Build history of the part. All positions in model axes, mm. Face numbers are marked on the shaded views. A direction names the side the tool comes from. Round coordinates to 2 decimals unless told otherwise and drop trailing zeros. Write each loop counter-clockwise with the first axis right and the second up, starting at its lowest first coordinate (ties: lowest second). Pieces come first, ordered by that corner, then holes. Notation, with made-up numbers: (86.25, 41) - (103.25, 41) arc R18 cw to (103.25, 56) - close; hole circle Ø5 at (78.5, 57). An arc over 180 degrees is marked (long way). Answer as a JSON object with one key per item and string values. Group by question number.
Item 1: Flat gauge pins, fed straight in: pin 1 (1.5 mm diameter, centred on x = 5.5, z = -0.5, fed in from +Y); pin 2 (1 mm diameter, centred on x = 5, y = 1, fed in from +Z). Where does each tip first touch, or does it go through?
Item 2: Slice it at A-A, the plane x = 7.75. List the corners of the cut face in (y, z), then the cut area to 3 significant figures.
Item 3: Probe line 1 (X direction, y = 1, z = -2.25); line 2 (X direction, y = -3, z = -0.25); line 3 (Y direction, x = 5.75, z = 0). List the from-to ranges inside material, lowest first. Write a range as from..to.
Item 4: Which spindle directions (+Z, -Z, +X, -X, +Y, -Y) get a long thin tool onto all of the face, cutting with end or side? Do the marked faces 1 and 2. Say none if no direction does.
from build123d import *

# Parameters (mm, degrees)
CUT_EXTRUDE_1_DEPTH = 1.53
CUT_EXTRUDE_1_TAPER = 10
FILLET_1_R          = 0.1


with BuildPart() as part:
    # Sketch 1 → Revolve 892 (revolve)
    with BuildSketch(Plane.XY, mode=Mode.PRIVATE) as revolve_892_sk:
        with BuildLine():
            Line((-2.162677546, 2.622032296), (-0.7, 2.75))
            Line((-0.7, 2.75), (-0.7, 3.25))
            Line((-0.7, 3.25), (0, 3.25))
            Line((0, 3.25), (0, 1.2))
            Line((0, 1.2), (0.5, 1.2))
            Line((0.5, 1.2), (0.5, 1.5))
            Line((0.5, 1.5), (10, 1.5))
            Line((10, 1.5), (10, 0))
            Line((10, 0), (-3.3, 0))
            ThreePointArc((-3.3, 0), (-3.234218103, 0.957402372), (-3.038108771, 1.896810531))
            ThreePointArc((-3.038108771, 1.896810531), (-2.713468973, 2.395917729), (-2.162677546, 2.622032296))
        make_face()
    revolve(revolve_892_sk.sketch.rotate(Axis((0, 0, 0), (1, 0, 0)), 90), axis=Axis((0, 0, 0), (1, 0, 0)))

    # Sketch 2 → Cut-Extrude 1 (cut)
    with BuildSketch(Plane(origin=(-3.3, 0, 0), x_dir=(0, 0, -1), z_dir=(1, 0, 0))):
        with BuildLine():
            Line((0.515, -1.85), (0.515, -0.815))
            ThreePointArc((0.515, -0.815), (0.602867966, -0.602867966), (0.815, -0.515))
            Line((0.815, -0.515), (1.85, -0.515))
            Line((1.85, -0.515), (1.85, 0.515))
            Line((1.85, 0.515), (0.815, 0.515))
            ThreePointArc((0.815, 0.515), (0.602867966, 0.602867966), (0.515, 0.815))
            Line((0.515, 0.815), (0.515, 1.85))
            Line((0.515, 1.85), (-0.515, 1.85))
            Line((-0.515, 1.85), (-0.515, 0.815))
            ThreePointArc((-0.515, 0.815), (-0.602867966, 0.602867966), (-0.815, 0.515))
            Line((-0.815, 0.515), (-1.85, 0.515))
            Line((-1.85, 0.515), (-1.85, -0.515))
            Line((-1.85, -0.515), (-0.815, -0.515))
            ThreePointArc((-0.815, -0.515), (-0.602867966, -0.602867966), (-0.515, -0.815))
            Line((-0.515, -0.815), (-0.515, -1.85))
            Line((-0.515, -1.85), (0.515, -1.85))
        make_face()
    extrude(amount=CUT_EXTRUDE_1_DEPTH, taper=CUT_EXTRUDE_1_TAPER, mode=Mode.SUBTRACT)

    # Fillet 1
    fillet_1_edges = [part.edges().sort_by_distance(p)[0] for p in [
        (0, 0, -1.2),
    ]]
    fillet(fillet_1_edges, radius=FILLET_1_R)


solid = part.part
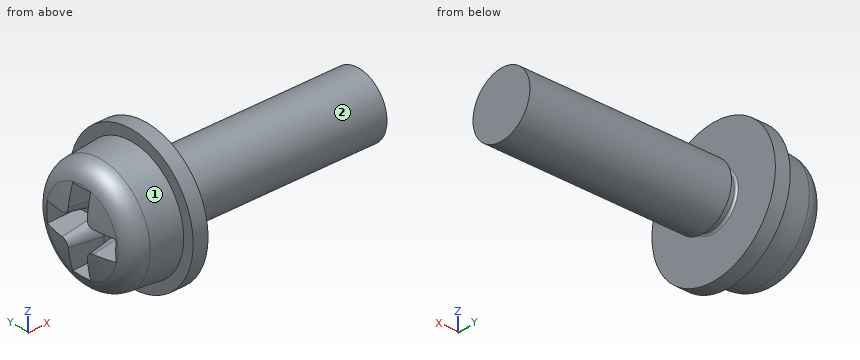
Geometry says:
{
 "1": {"pin 1": "stops at y = 1.5", "pin 2": "stops at z = 1.41"},
 "2": {"outline": "circle Ø3 at (0, 0)", "area": "7.07 mm^2"},
 "3": {"line 1": "x = -2.62..0", "line 2": "x = -0.7..0", "line 3": "y = -1.5..1.5"},
 "4": {"face 1": "-X", "face 2": "+X"}
}
